from build123d import *

# Parameters (mm, degrees)
SALIENTE_EXTRUIR1_DEPTH           = 2
DI_METRO_DE_TALADRO_4_0_4_1_D     = 4
DI_METRO_DE_TALADRO_4_0_4_1_DEPTH = 3.323811401
CROQUIS4_R                        = 4.25
SALIENTE_EXTRUIR2_DEPTH           = 7
SALIENTE_EXTRUIR3_DEPTH           = 15
CORTAR_EXTRUIR1_DEPTH             = 15
CROQUIS7_R                        = 6.125
SALIENTE_EXTRUIR4_DEPTH           = 2


with BuildPart() as part:
    # Croquis1 → Saliente-Extruir1 (new body)
    with BuildSketch(Plane(origin=(-45.591866133, -7.28172098, 0), x_dir=(0.15771642640636402, -0.9874844448605792, 0), z_dir=(-0.9874844448605792, -0.15771642640636402, 0))):
        with BuildLine():
            Line((51.04106459, 0), (42.54106459, 0))
            Line((42.54106459, 0), (42.54106459, -1))
            ThreePointArc((42.54106459, -1), (46.79106459, -5.25), (51.04106459, -1))
            Line((51.04106459, -1), (51.04106459, 0))
        make_face()
    extrude(amount=-SALIENTE_EXTRUIR1_DEPTH)

    # Diámetro de taladro Ø4.0 (4)1
    with Locations(Plane(origin=(-43.616897243, -6.966288127, 0), x_dir=(0, 0, -1), z_dir=(0.9874844448605791, 0.15771642640636402, 0))):
        with Locations((1, -46.79106459)):
            Hole(DI_METRO_DE_TALADRO_4_0_4_1_D / 2, depth=DI_METRO_DE_TALADRO_4_0_4_1_DEPTH)

    # Croquis4 → Saliente-Extruir2 (add)
    with BuildSketch(Plane(origin=(0, 0, 0), x_dir=(-1, 0, 0), z_dir=(0, 0, -1))):
        with Locations(Location((37.224662193, -53.329452995, 0), (0, 0, 67.316665151))):
            Circle(CROQUIS4_R)
    extrude(amount=-SALIENTE_EXTRUIR2_DEPTH)

    # Croquis5 → Saliente-Extruir3 (add)
    with BuildSketch(Plane.XY.offset(7)):
        with BuildLine():
            Line((-39.623054784, -49.408647851), (-37.894957006, -49.132644104))
            ThreePointArc((-37.894957006, -49.132644104), (-33.027853303, -52.659158183), (-36.554367381, -57.526261886))
            Line((-36.554367381, -57.526261886), (-38.28246516, -57.802265632))
            Line((-38.28246516, -57.802265632), (-39.623054784, -49.408647851))
        make_face()
    extrude(amount=SALIENTE_EXTRUIR3_DEPTH)

    # Croquis6 → Cortar-Extruir1 (cut)
    with BuildSketch(Plane.XY.offset(22)):
        Polygon((-38.724725024, -50.277844976), (-39.712209469, -50.435561402), (-38.687052697, -56.854210294), (-37.699568252, -56.696493867), align=None)
    extrude(amount=-CORTAR_EXTRUIR1_DEPTH, mode=Mode.SUBTRACT)

    # Croquis7 → Saliente-Extruir4 (add)
    with BuildSketch(Plane(origin=(0, 0, 7), x_dir=(-1, 0, 0), z_dir=(0, 0, -1))):
        with Locations((37.21095217, -53.415293358)):
            Circle(CROQUIS7_R)
    extrude(amount=SALIENTE_EXTRUIR4_DEPTH)


solid = part.part
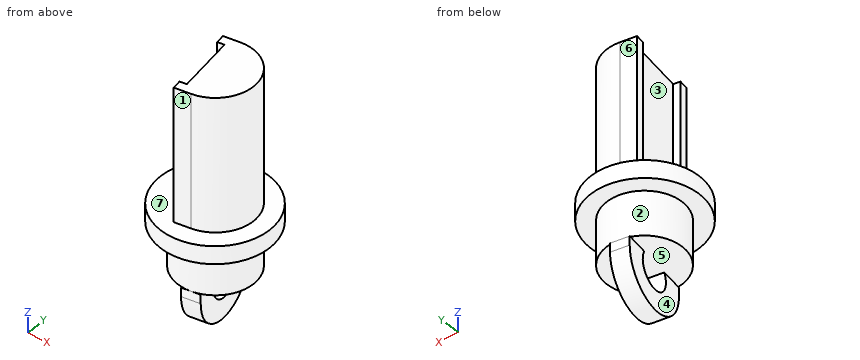
Input: part model. Units: mm. Frame: model coordinates. Face numbers are marked on the shaded views. A direction names the side the tool comes from. Coordinates: 2 decimals unless noted, no trailing zeros. Order: outer loops, then holes, each group sorted by start corner. A loop starts at its lowest first (then second) coordinate and runs counter-clockwise, first axis right, second up. Notation, with made-up numbers: M 56,51 L 77,51 A12 cw 77,71 Z; hole C -40,62.25 d2. An arc over 180 degrees is marked long. One line per question, with ' | ' between items.
Item 1: Ray query, line 1 along Z through (x, y) = (-40.25, -52.25); line 2 along Z through (x, y) = (-37, -55); line 3 along Z through (x, y) = (-35.5, -53.75). Return the intervals inside material, ascending.
Geometry results:
line 1: z = 0 to 7 | line 2: z = -4.9 to -2.08, 0 to 22 | line 3: z = 0 to 22
Item 2: Pin query (flat end, axial travel): pin 1 (5 mm diameter, centred on y = -53, z = -2, fed in from +X); pin 2 (1 mm diameter, centred on y = -56, z = 3, fed in from +X); pin 3 (1 mm diameter, centred on x = -33.5, z = 2.5, fed in from +Y). Return the tip coordinate at first contact, or that it passes through.
Geometry results:
pin 1: stops at x = -32.97 | pin 2: stops at x = -33.57 | pin 3: stops at y = -50.56
Item 3: Section B-B (z = -2.25). Output: boundary loops of the cut face in (x, y), then the cut area to 3 significant figures.
Geometry results:
outline: M -38.85,-49.48 L -38.46,-51.95 L -36.48,-51.63 L -36.88,-49.16 Z; M -37.97,-55.03 L -37.57,-57.5 L -35.6,-57.18 L -35.99,-54.71 Z | area: 10.0 mm^2
Item 4: Section C-C (x = -35). Output: boundary loops of the cut face in (y, z).
Geometry results:
outline: M -59.13,5 L -56.95,5 L -56.95,0 L -49.71,0 L -49.71,5 L -47.7,5 L -47.7,7 L -49.71,7 L -49.71,22 L -56.95,22 L -56.95,7 L -59.13,7 Z
Item 5: Draft query along Y for the marked faces 1, 2 and 3. Return one class per face: released by +Y, released by -Y, zero draft, split by the parting line, or undercut.
Geometry results:
face 1: released by -Y | face 2: split by the parting line | face 3: undercut
Item 6: Reachability of the marked faces 4, 5, 6 and 7 from +Z, -Z, +X, -X, +Y, -Y: full face, straight path, thin tool, end or side. Return the list, or none.
Geometry results:
face 4: -Z, -X, -Y | face 5: none | face 6: +Z, -X, +Y | face 7: +Z
Item 7: Section A-A (z = 19). Output: boundary loops of the cut face in (x, y), then the cut area to 3 significant figures.
Geometry results:
outline: M -39.62,-49.41 L -39.47,-50.4 L -38.72,-50.28 L -37.7,-56.7 L -38.44,-56.81 L -38.28,-57.8 L -36.55,-57.53 A4.25 ccw -37.89,-49.13 Z | area: 38.4 mm^2
Item 8: Section D-D (y = -48.5). Output: boundary loops of the cut face in (x, z).
Geometry results:
outline: M -40.87,5 L -33.56,5 L -33.56,7 L -40.87,7 Z
